Geometry: final body of the model. Coordinates: model frame, mm. A direction names the side the tool comes from. Coordinates: 2 decimals unless noted, no trailing zeros. Write each loop counter-clockwise with the first axis right and the second up, starting at its lowest first coordinate (ties: lowest second). Pieces come first, ordered by that corner, then holes.
from build123d import *

# Parameters (mm, degrees)
BOSS_EXTRUDE1_DEPTH = 7.5
CUT_EXTRUDE1_DEPTH  = 5.5
CUT_EXTRUDE2_START  = -9.5
CUT_EXTRUDE2_DEPTH  = 5.5
SKETCH3_R           = 4.000000000000006
CUT_EXTRUDE3_DEPTH  = 55.1894823743501
CUT_EXTRUDE3_DRAFT  = 10.000000000000002
FILLET1_R           = 2.5
CUT_EXTRUDE4_START  = -2
CUT_EXTRUDE4_DEPTH  = 2
FILLET2_R           = 10
FILLET5_R           = 1
FILLET3_R           = 1


with BuildPart() as part:
    # Sketch1 → Boss-Extrude1 (new, symmetric)
    with BuildSketch(Plane.XY):
        with BuildLine():
            Line((-5.249999999999999, 12), (-5.249999999999999, -5.25))
            Line((-5.249999999999999, -5.25), (50, -5.25))
            Line((50, -5.25), (50, -2.2500000000000004))
            Line((50, -2.2500000000000004), (5.250000000000001, -2.2500000000000004))
            Line((5.250000000000001, -2.2500000000000004), (5.249999999999999, 12))
            ThreePointArc((5.249999999999999, 12), (3.2e-16, 17.25), (-5.249999999999999, 12))
        make_face()
        with BuildLine():
            Line((1.2499999999999998, 12), (1.2500000000000002, 0))
            ThreePointArc((1.2500000000000002, 0), (-2.3e-16, -1.2500000000000002), (-1.2500000000000002, 0))
            Line((-1.2500000000000002, 0), (-1.2499999999999998, 12))
            ThreePointArc((-1.2499999999999998, 12), (8e-17, 13.25), (1.2499999999999998, 12))
        make_face(mode=Mode.SUBTRACT)
    extrude(amount=BOSS_EXTRUDE1_DEPTH, both=True)

    # Sketch2 → Cut-Extrude1 (cut)
    with BuildSketch(Plane.XY.offset(7.5)):
        with BuildLine():
            Line((-5.249999999999999, 12), (-5.249999999999996, -2.2500000000000018))
            Line((-5.249999999999996, -2.2500000000000018), (5.250000000000001, -2.2500000000000004))
            Line((5.250000000000001, -2.2500000000000004), (5.249999999999999, 12))
            ThreePointArc((5.249999999999999, 12), (3.2e-16, 17.25), (-5.249999999999999, 12))
        make_face()
    extrude(amount=-CUT_EXTRUDE1_DEPTH, mode=Mode.SUBTRACT)

    # Sketch2<2> → Cut-Extrude2 (cut)
    with BuildSketch(Plane.XY.offset(7.5).offset(CUT_EXTRUDE2_START)):
        with BuildLine():
            Line((-5.249999999999999, 12), (-5.249999999999996, -2.2500000000000018))
            Line((-5.249999999999996, -2.2500000000000018), (5.250000000000001, -2.2500000000000004))
            Line((5.250000000000001, -2.2500000000000004), (5.249999999999999, 12))
            ThreePointArc((5.249999999999999, 12), (3.2e-16, 17.25), (-5.249999999999999, 12))
        make_face()
    extrude(amount=-CUT_EXTRUDE2_DEPTH, mode=Mode.SUBTRACT)


with BuildPart() as cut_extrude3_tool:
    # Sketch3 → Cut-Extrude3 (with draft: the straight prism first)
    with BuildSketch(Plane(origin=(0, -2.2500000000000004, 0), x_dir=(1, 0, 0), z_dir=(0, 1, 0))):
        with Locations((30, 0)):
            Circle(SKETCH3_R)
    extrude(amount=-CUT_EXTRUDE3_DEPTH)
    # Cut-Extrude3: the draft: its side faces are tilted about the plane it starts from
    cut_extrude3_sides = [cut_extrude3_tool.faces().sort_by_distance(p)[0] for p in [
        (26, -29.844741187, 0),
    ]]
    draft(cut_extrude3_sides, Plane(origin=(0, -2.2500000000000004, 0), x_dir=(1, 0, 0), z_dir=(0, 1, 0)), CUT_EXTRUDE3_DRAFT)


with BuildPart() as part_1:
    add(part.part)

    # Cut-Extrude3: cut by cut_extrude3_tool
    add(cut_extrude3_tool.part, mode=Mode.SUBTRACT)

    # Fillet1
    fillet1_edges = [part_1.edges().sort_by_distance(p)[0] for p in [
        (50, -3.75, 7.5),
        (-5.249999999999999, -3.75, 7.5),
        (-5.249999999999999, -3.75, -7.5),
        (50, -3.75, -7.5),
    ]]
    fillet(fillet1_edges, radius=FILLET1_R)

    # Sketch4 → Cut-Extrude4 (cut)
    with BuildSketch(Plane(origin=(0, -2.2500000000000004, 0), x_dir=(1, 0, 0), z_dir=(0, 1, 0)).offset(CUT_EXTRUDE4_START)):
        with BuildLine():
            Line((5.250000000000001, 2.0000000000000018), (-5.249999999999996, 2.0000000000000018))
            Line((-5.249999999999996, 2.0000000000000018), (-5.249999999999996, 4.999999999999997))
            ThreePointArc((-5.249999999999996, 4.999999999999997), (-4.517766952966367, 6.767766952966371), (-2.7499999999999956, 7.5))
            Line((-2.7499999999999956, 7.5), (5.250000000000003, 7.5))
            Line((5.250000000000003, 7.5), (5.250000000000001, 2.0000000000000018))
        make_face()
    extrude(amount=CUT_EXTRUDE4_DEPTH, mode=Mode.SUBTRACT)

    # Fillet2
    # the kernel refuses this fillet: 10 mm, written as the material it adds along each edge
    with BuildSketch(Plane(origin=(5.250000000000003, -4.25, -7.5), x_dir=(-1.168e-13, 1, 0), z_dir=(-3.2e-16, 0, 1))) as fillet2_piece_1_section:
        with BuildLine():
            CenterArc((10.0000000000007, 5.99999999999948), FILLET2_R, 179.99999999999332, 36.869897645847004)
            Line((7.0077e-13, 6.000000000000648), (0, 0))
            Line((0, 0), (2.0000000000003118, 0))
        make_face()
    fillet2_piece_1 = extrude(amount=20.500000000001616, mode=Mode.PRIVATE)
    fillet2_piece_1 = split(fillet2_piece_1, bisect_by=Plane(origin=(2.41860221548833, -3.7558066464660698, 2), z_dir=(0, 0, -1)), keep=Keep.TOP, mode=Mode.PRIVATE)
    add(fillet2_piece_1)

    # Fillet5
    fillet5_edges = [part_1.edges().sort_by_distance(p)[0] for p in [
        (5.250000000000002, -2.2500000000000004, -4.750000000000001),
    ]]
    fillet(fillet5_edges, radius=FILLET5_R)

    # Fillet3
    # the kernel refuses this fillet: 1 mm, written as the material it adds along each edge
    with BuildSketch(Plane(origin=(-0.7499999999989999, 5.750000000001, -2.0000000000000018), x_dir=(0.5749595745759393, -0.8181818181819093, 0), z_dir=(0.8181818181819093, 0.5749595745759393, 0))) as fillet3_piece_1:
        with BuildLine():
            CenterArc((10 - FILLET3_R, FILLET3_R), FILLET3_R, 270, 90)
            Line((10 - FILLET3_R, 0), (10, 0))
            Line((10, 0), (10, FILLET3_R))
        make_face()
    revolve(axis=Axis((-0.7499999999989999, 5.750000000001, -2.0000000000000018), (0, 0, -1)), revolution_arc=35.0968012275825)
    with BuildSketch(Plane(origin=(-0.7500000000006111, -4.25, -2.0000000000000018), x_dir=(0, 0, -1), z_dir=(-1, 0, 0))) as fillet3_piece_2:
        with BuildLine():
            CenterArc((FILLET3_R, -FILLET3_R), FILLET3_R, 90, 90)
            Line((0, -FILLET3_R), (0, 0))
            Line((0, 0), (FILLET3_R, 0))
        make_face()
    extrude(amount=4.4999999999993845)
    with BuildSketch(Plane(origin=(5.574555320336334, -3.250000000000001, -2.0000000000000018), x_dir=(-0.5749595745759413, 0.818181818181908, 0), z_dir=(-0.818181818181908, -0.5749595745759413, 0))) as fillet3_piece_3_section:
        with BuildLine():
            CenterArc((1.0000000000000002 + FILLET3_R, FILLET3_R), FILLET3_R, 180, 90)
            Line((1.0000000000000002 + FILLET3_R, 0), (1.0000000000000002, 0))
            Line((1.0000000000000002, 0), (1.0000000000000002, FILLET3_R))
        make_face()
    fillet3_piece_3 = revolve(axis=Axis((5.574555320336334, -3.250000000000001, -2.0000000000000018), (0, 0, -1)), revolution_arc=178.34499823253051, mode=Mode.PRIVATE)
    fillet3_piece_3 = split(fillet3_piece_3, bisect_by=Plane(origin=(5.250000000000001, -2.3158219875897332, -2.423725348187279), z_dir=(-1, -1.2e-16, 0)), keep=Keep.TOP, mode=Mode.PRIVATE)
    add(fillet3_piece_3)
    with BuildSketch(Plane(origin=(5.574555320336334, -3.250000000000001, -2.0000000000000018), x_dir=(-0.5749595745759413, 0.818181818181908, 0), z_dir=(-0.818181818181908, -0.5749595745759413, 0))) as fillet3_piece_4_section:
        with BuildLine():
            CenterArc((1.0000000000000002 + FILLET3_R, FILLET3_R), FILLET3_R, 180, 90)
            Line((1.0000000000000002 + FILLET3_R, 0), (1.0000000000000002, 0))
            Line((1.0000000000000002, 0), (1.0000000000000002, FILLET3_R))
        make_face()
    fillet3_piece_4 = revolve(axis=Axis((5.574555320336334, -3.250000000000001, -2.0000000000000018), (0, 0, -1)), revolution_arc=178.34499823253051, mode=Mode.PRIVATE)
    fillet3_piece_4 = split(fillet3_piece_4, bisect_by=Plane(origin=(5.333721819231152, -2.2500000000000004, -2.422839116405143), z_dir=(1.3e-16, -1, 0)), keep=Keep.TOP, mode=Mode.PRIVATE)
    add(fillet3_piece_4)


solid = part_1.part
Item 1: Material intervals for probe 1 along X at (y, z) = (8.5, -0.75); probe 2 along Y at (x, z) = (33, 4.25); probe 3 along Z at (x, y) = (2, 9), sorted ascending.
Derived:
probe 1: x = -5.25 to -1.25, 1.25 to 5.25
probe 2: y = -5.25 to -2.25
probe 3: z = -2 to 2
Item 2: Section B-B, the plane y = 8.5. Output: boundary loops of the cut face in (x, z), plus the area to 3 significant figures.
Derived:
outline: (-5.25, -2) - (-1.25, -2) - (-1.25, 2) - (-5.25, 2) - close; (1.25, -2) - (5.25, -2) - (5.25, 2) - (1.25, 2) - close
area: 32.0 mm2
Item 3: Section D-D, the plane x = 12. Output: boundary loops of the cut face in (y, z).
Derived:
outline: (-5.25, -7.5) - (-2.25, -7.5) - (-2.25, 7.5) - (-5.25, 7.5) - close
Item 4: Pull-direction query (Y, two-part tool) for faces 6 (the flat face through (-2, 8, 2)), 7 (the flat face through (-3, -4.25, -5)), 8 (the cylindrical face through (0.03, -1.25, 0.03)); classes: released by +Y, released by -Y, zero draft, split by the parting line, or undercut.
Derived:
face 6: zero draft
face 7: released by +Y
face 8: undercut
Item 5: Set-up query: faces 1 (the flat face through (-2, 7, -2)), 2 (the cylindrical face through (49, -4, 7)), 3 (the flat face through (1.25, 6, 0)), 4 (the flat face through (5.25, 5, 0)), 5 (the cylindrical face through (0.12, 17.25, 0.03)). Return all of +Z, -Z, +X, -X, +Y, -Y with unobstructed straight access to the full face (end or side cutting, diameter ignored); none if empty.
Derived:
face 1: -Z, -X, +Y
face 2: +Z, +X, +Y, -Y
face 3: +Z, -Z
face 4: +Z, -Z, +X, +Y
face 5: +Z, -Z, +Y
Item 6: Section C-C, the plane x = 30. Output: boundary loops of the cut face in (y, z), plus the area to 3 significant figures.
Derived:
outline: (-5.25, -7.5) - (-2.25, -7.5) - (-2.25, -4) - (-5.25, -4.53) - close; (-5.25, 4.53) - (-2.25, 4) - (-2.25, 7.5) - (-5.25, 7.5) - close
area: 19.4 mm2
Item 7: Pin query (flat end, axial travel): pin 1 (6 mm diameter, centred on y = 1.5, z = 0.5, fed in from +X); pin 2 (3.5 mm diameter, centred on x = -2, z = -4.5, fed in from +Y); pin 3 (3 mm diameter, centred on x = 1.5, y = 6, fed in from +Z). Return the tip coordinate at first contact, or that it passes through.
Derived:
pin 1: stops at x = 5.25
pin 2: stops at y = -4.22
pin 3: stops at z = 2
Item 8: Section A-A, the plane z = 0. Output: boundary loops of the cut face in (x, y).
Derived:
outline: (-5.25, -5.25) - (25.47, -5.25) - (26, -2.25) - (5.25, -2.25) - (5.25, 12) arc R5.25 ccw to (-5.25, 12) - close; (34, -2.25) - (34.53, -5.25) - (50, -5.25) - (50, -2.25) - close; hole (-1.25, 0) arc R1.25 ccw to (1.25, 0) - (1.25, 12) arc R1.25 ccw to (-1.25, 12) - close
